Can you work these out from the model? Positions are in its coordinate system, mm. A direction names the side the tool comes from. Coordinates: 2 decimals unless noted, no trailing zeros. Order: outer loops, then holes, each group sorted by start corner. A loop starts at its lowest first (then second) coordinate and runs counter-clockwise, first axis right, second up. Notation, with made-up numbers: (50.5, -18) -> (61.5, -18) arc R22 cw to (61.5, 15) -> close; hole circle Ø6 at (-23, -33). An arc over 180 degrees is marked (long way). Answer in a Markdown table with one row per item.
```python
from build123d import *

# Parameters (mm, degrees)
EXTRUDE_1_DEPTH     = 2
CUT_EXTRUDE_2_DEPTH = 1
SKETCH_4_W          = 133.19
SKETCH_4_H          = 55
SKETCH_4_W_2        = 130.19
SKETCH_4_H_2        = 53.761168256
EXTRUDE_2_DEPTH     = 4


with BuildPart() as part:
    # 草图1 → 凸台-拉伸1 (new body)
    with BuildSketch(Plane.XY):
        with BuildLine():
            Line((-64, 29), (64, 29))
            ThreePointArc((64, 29), (68.242640687, 27.242640687), (70, 23))
            Line((70, 23), (70, -23))
            ThreePointArc((70, -23), (68.242640687, -27.242640687), (64, -29))
            Line((64, -29), (-64, -29))
            ThreePointArc((-64, -29), (-68.242640687, -27.242640687), (-70, -23))
            Line((-70, -23), (-70, 23))
            ThreePointArc((-70, 23), (-68.242640687, 27.242640687), (-64, 29))
        make_face()
    extrude(amount=EXTRUDE_1_DEPTH)

    # 草图3 → 切除-拉伸2 (cut)
    with BuildSketch(Plane.XY.offset(2)):
        with BuildLine():
            ThreePointArc((1.846153846, -7.217800499), (3.411683714, -7.465870337), (4.81172184, -6.722690911))
            ThreePointArc((4.81172184, -6.722690911), (6.276265295, -4.837971823), (7.338817992, -2.700675555))
            ThreePointArc((7.338817992, -2.700675555), (4.117591942, 0.931901262), (6.77351325, 4.99613472))
            ThreePointArc((6.77351325, 4.99613472), (6.502838049, 5.308433669), (6.211306836, 5.601359))
            ThreePointArc((6.211306836, 5.601359), (4.080647383, 6.637601762), (1.7375, 6.286647199))
            ThreePointArc((1.7375, 6.286647199), (0, 5.889575695), (-1.7375, 6.286647199))
            ThreePointArc((-1.7375, 6.286647199), (-4.080647383, 6.637601762), (-6.211306835, 5.601359))
            ThreePointArc((-6.211306835, 5.601359), (-7.674507441, 3.461224238), (-8.098236156, 0.903571645))
            ThreePointArc((-8.098236156, 0.903571645), (-7.135696802, -3.20291287), (-4.81172184, -6.722690911))
            ThreePointArc((-4.81172184, -6.722690911), (-3.411683714, -7.465870337), (-1.846153846, -7.217800499))
            ThreePointArc((-1.846153846, -7.217800499), (0, -6.766281297), (1.846153846, -7.217800499))
        make_face()
        with BuildLine():
            ThreePointArc((0.506524653, 7.007542389), (2.728267025, 8.585588777), (3.423600981, 11.22052336))
            ThreePointArc((3.423600981, 11.22052336), (0.540506505, 9.788938293), (-0.354358224, 6.696869944))
            ThreePointArc((-0.354358224, 6.696869944), (0.070150926, 6.868644721), (0.506524653, 7.007542389))
        make_face()
    extrude(amount=-CUT_EXTRUDE_2_DEPTH, mode=Mode.SUBTRACT)

    # 草图4 → 凸台-拉伸2 (add)
    with BuildSketch(Plane(origin=(0, 0, 0), x_dir=(-1, 0, 0), z_dir=(0, 0, -1))):
        Rectangle(SKETCH_4_W, SKETCH_4_H)
        Rectangle(SKETCH_4_W_2, SKETCH_4_H_2, mode=Mode.SUBTRACT)
    extrude(amount=EXTRUDE_2_DEPTH)


solid = part.part
```
(1) Suppose I cut it at D-D (y = 2.5). Please give me the cut outline in (x, z) (3 decimals).
Response values:
| item | result |
|---|---|
| outline | (-70, 0) -> (-66.595, 0) -> (-66.595, -4) -> (-65.095, -4) -> (-65.095, 0) -> (65.095, 0) -> (65.095, -4) -> (66.595, -4) -> (66.595, 0) -> (70, 0) -> (70, 2) -> (4.316, 2) -> (4.316, 1) -> (-7.97, 1) -> (-7.97, 2) -> (-70, 2) -> close |
(2) Suppose I cut it at B-B (x = 9). Please give me the cut outline in (y, z).
Response values:
| item | result |
|---|---|
| outline | (-29, 0) -> (-27.5, 0) -> (-27.5, -4) -> (-26.88, -4) -> (-26.88, 0) -> (26.88, 0) -> (26.88, -4) -> (27.5, -4) -> (27.5, 0) -> (29, 0) -> (29, 2) -> (-29, 2) -> close |
(3) Suppose I cut it at C-C (y = -20). Please give me the cut outline in (x, z) (3 decimals), and give its area (3 significant figures).
Response values:
| item | result |
|---|---|
| outline | (-70, 0) -> (-66.595, 0) -> (-66.595, -4) -> (-65.095, -4) -> (-65.095, 0) -> (65.095, 0) -> (65.095, -4) -> (66.595, -4) -> (66.595, 0) -> (70, 0) -> (70, 2) -> (-70, 2) -> close |
| area | 292 mm2 |
(4) We'd pull the mould along X, two halves only. Please class faces 1 (the flat face through (-66.595, 0, -2)), 2 (the flat face through (-65.095, 0, -2)), 3 (the flat face through (1, -27.5, -2)): +X half, -X half, draft (parallel to the pull), parting line (faces both ways), or undercut.
Response values:
| item | result |
|---|---|
| face 1 | -X half |
| face 2 | undercut |
| face 3 | draft |
(5) Suppose I cut it at A-A (z = -1.4). Please give me the cut outline in (x, y) (3 decimals), and give its area (3 significant figures).
Response values:
| item | result |
|---|---|
| outline | (-66.595, -27.5) -> (66.595, -27.5) -> (66.595, 27.5) -> (-66.595, 27.5) -> close; hole (-65.095, -26.881) -> (65.095, -26.881) -> (65.095, 26.881) -> (-65.095, 26.881) -> close |
| area | 326 mm2 |
(6) On a 3-axis mill with a long thin cutter (end or side, diameter ignored), from which of +Z, -Z, +X, -X, +Y, -Y can I reach the whole of each face in a straight line? I mean faces 4 (the cylindrical face through (-68.289, 27.196, 0.986)), 5 (the cylindrical face through (2.706, 8.554, 1.507)), 6 (the flat face through (66.595, 0, -2)), 7 (the cylindrical face through (68.289, -27.196, 0.986)), 8 (the flat face through (1, -26.881, -2)). Say none if no direction works.
Response values:
| item | result |
|---|---|
| face 4 | +Z, -Z, -X, +Y |
| face 5 | +Z |
| face 6 | -Z, +X, +Y, -Y |
| face 7 | +Z, -Z, +X, -Y |
| face 8 | -Z |
(7) Will these pins go through, and if not, where does the flat tip stop? pin 1 Ø1.2 at (y, z) = (-2, -2) entering from +X (3 decimals); pin 2 Ø8 at (x, y) = (5.5, -6.5) entering from -Z; pin 3 Ø1.2 at (x, z) = (28.5, -2) entering from +Y.
Response values:
| item | result |
|---|---|
| pin 1 | x = 66.595 |
| pin 2 | z = 0 |
| pin 3 | y = 27.5 |
(8) I need wall thicknesses on line 1 (X direction, y = -5.5, z = -1.85) (3 decimals); line 2 (Y direction, x = 46, z = -0.95); line 3 (Z direction, x = -25.5, y = -23). Which ranges of each line are inside material? Lowest first, please. Write a range as [from, to].
Response values:
| item | result |
|---|---|
| line 1 | [-66.595, -65.095], [65.095, 66.595] |
| line 2 | [-27.5, -26.88], [26.88, 27.5] |
| line 3 | [0, 2] |
